```python
from build123d import *

# Parameters (mm, degrees)
F1_DEPTH = 600
F3_DEPTH = 50.001
F5_DEPTH = 50.001


with BuildPart() as f1:
    # F0 (on Top) → F1 (new body)
    with BuildSketch(Plane.XY):
        Polygon((0, 50), (0, 0), (50, 0), (50, 8), (8, 8), (8, 50), align=None)
    extrude(amount=F1_DEPTH)

    # F2 (on face) → F3 (cut, through all)
    with BuildSketch(Plane(origin=(0, 0, 0), x_dir=(0, -1, 0), z_dir=(-1, 0, 0))):
        Polygon((-50, 550), (0, 600), (-50, 600), align=None)
    extrude(amount=-F3_DEPTH, mode=Mode.SUBTRACT)

    # F4 (on face) → F5 (cut, through all)
    with BuildSketch(Plane(origin=(0, 0, 0), x_dir=(0, -1, 0), z_dir=(-1, 0, 0))):
        Polygon((-50, 0), (0, 0), (-50, 50), align=None)
    extrude(amount=-F5_DEPTH, mode=Mode.SUBTRACT)


solid = f1.part
```
CAD build for the part. Positions are in the model's coordinates, mm. A direction names the side the tool comes from. Coordinates: 2 decimals unless noted, no trailing zeros. Write each loop counter-clockwise with the first axis right and the second up, starting at its lowest first coordinate (ties: lowest second). Pieces come first, ordered by that corner, then holes. Notation, with made-up numbers: (28.25, -14) -> (45.25, -14) arc R29 ccw to (45.25, 9) -> close; hole circle Ø1 at (66, 9). An arc over 180 degrees is marked (long way). Return JSON: item names as keys, results as strings. Group by question number.
Q1. Which spindle directions (+Z, -Z, +X, -X, +Y, -Y) get a long thin tool onto all of the face, cutting with end or side? Do faces 1 (the face through (29, 8, 296)), 2 (the face through (2, 14, 14)). Say none if no direction does.
Q2. Flat gauge pins, fed straight in: pin 1 (8 mm diameter, centred on x = 29.5, z = 374.5, fed in from +Y); pin 2 (10 mm diameter, centred on y = 37.5, z = 371, fed in from +X); pin 3 (10 mm diameter, centred on x = 31.5, y = 5.5, fed in from +Z). Where does each tip first touch, or does it go through?
Q3. Drill centre lines: line 1 (Y direction, x = 9.5, z = 304); line 2 (Z direction, x = 29, y = 7). Where is each one in solid material? Low to high.
Q4. Cut at C-C, the plane x = 35. Give the cut face in (y, z).
Q5. Cut at B-B, the plane y = 28. Give the cut face in (x, z).
Q6. Cut at A-A, the plane z = 139. Give the cut face in (x, y), then the cut area to 3 significant figures.
Returned:
{
 "1": {"face 1": "+Z, -Z, +X, +Y", "face 2": "-Z, +X, -X, +Y"},
 "2": {"pin 1": "stops at y = 8", "pin 2": "stops at x = 8", "pin 3": "stops at z = 599.5"},
 "3": {"line 1": "y = 0 to 8", "line 2": "z = 7 to 593"},
 "4": {"outline": "(0, 0) -> (8, 8) -> (8, 592) -> (0, 600) -> close"},
 "5": {"outline": "(0, 28) -> (8, 28) -> (8, 572) -> (0, 572) -> close"},
 "6": {"outline": "(0, 0) -> (50, 0) -> (50, 8) -> (8, 8) -> (8, 50) -> (0, 50) -> close", "area": "736 mm2"}
}
